```python
from build123d import *

# Parameters (mm, degrees)
DODANIE_WYCI_GNI_CIE1_DEPTH = 9.5


with BuildPart() as part:
    # Szkic1 → Dodanie-wyci_gni_cie1 (new body)
    with BuildSketch(Plane(origin=(0, 0, 0), x_dir=(1, 0, 0), z_dir=(0, 1, 0))):
        with BuildLine():
            ThreePointArc((8, 0), (-3.464101615, -7.211102551), (-5, 6.244997998))
            Line((-5, 6.244997998), (-5, 8))
            Line((-5, 8), (-12.25, 8))
            Line((-12.25, 8), (-12.25, -19))
            Line((-12.25, -19), (12.25, -19))
            Line((12.25, -19), (12.25, 8))
            Line((12.25, 8), (5, 8))
            Line((5, 8), (5, 6.244997998))
            ThreePointArc((5, 6.244997998), (7.211102551, 3.464101615), (8, 0))
        make_face()
        with BuildLine():
            ThreePointArc((5, 0), (0, -5), (-5, 0))
            Line((-5, 0), (-5, 6.244997998))
            ThreePointArc((-5, 6.244997998), (-3.464101615, -7.211102551), (8, 0))
            ThreePointArc((8, 0), (7.211102551, 3.464101615), (5, 6.244997998))
            Line((5, 6.244997998), (5, 0))
        make_face()
    extrude(amount=DODANIE_WYCI_GNI_CIE1_DEPTH)


solid = part.part
```
Model file for the job. Use its own axes, mm. Round coordinates to 2 decimals unless told otherwise and drop trailing zeros. Write each loop counter-clockwise with the first axis right and the second up, starting at its lowest first coordinate (ties: lowest second). Pieces come first, ordered by that corner, then holes. Notation, with made-up numbers: M 56,5.25 L 74,5.25 A21 ccw 74,23.25 Z; hole C -4.75,-10 d11. An arc over 180 degrees is marked long. Put each result on its own line as item: value.
Item 1: Cut at C-C (x = 4). List the corners of the cut face in (y, z), and give its area (3 significant figures).
Responses:
outline: M 0,3 L 9.5,3 L 9.5,19 L 0,19 Z
area: 152 mm²
Item 2: Probe L1, parallel to X at y = 6.5, z = -4.75; L2, parallel to X at y = 1.25, z = 4.5; L3, parallel to Z at x = 2.75, y = 5.5. List the from-to ranges inside material, lowest first. Write a range as from..to.
Responses:
L1: -12.25..-5, 5..12.25
L2: -12.25..-2.18, 2.18..12.25
L3: 4.18..19
Item 3: Cut at A-A (z = -1.25). List the corners of the cut face in (x, y), and give its area (3 significant figures).
Responses:
outline: M -12.25,0 L -5,0 L -5,9.5 L -12.25,9.5 Z; M 5,0 L 12.25,0 L 12.25,9.5 L 5,9.5 Z
area: 138 mm²
Item 4: Mould opens along X. For faces 1 (the flat face through (12.25, 5, 6)), 2 (the flat face through (-0.2, 9.5, 5.3)), 3 (the flat face through (-5, 5, -4)), 4 (the flat face through (5, 5, -4)) say: +X half, -X half, draft (parallel to the pull), parting line (faces both ways), or undercut.
Responses:
face 1: +X half
face 2: draft
face 3: undercut
face 4: undercut
Item 5: Cut at B-B (y = 3). List the corners of the cut face in (x, z).
Responses:
outline: M -12.25,-8 L -5,-8 L -5,0 A5 cw 5,0 L 5,-8 L 12.25,-8 L 12.25,19 L -12.25,19 Z
Item 6: Cut at D-D (x = 0). List the corners of the cut face in (y, z), and give its area (3 significant figures).
Responses:
outline: M 0,5 L 9.5,5 L 9.5,19 L 0,19 Z
area: 133 mm²
